Read the model definition and answer for the solid it produces. Units are mm, in the model's axes. Face numbers are marked on the shaded views. A direction names the side the tool comes from. Give positions to 0.01 mm unless a question says otherwise; leave off trailing zeros. Write each loop counter-clockwise with the first axis right and the second up, starting at its lowest first coordinate (ties: lowest second). Pieces come first, ordered by that corner, then holes. Notation, with made-up numbers: M -14.75,56 L 23.25,56 A29 ccw 23.25,89 Z; hole C 83.5,14.5 d2. An arc over 180 degrees is marked long. Put each result on its own line as item: value.
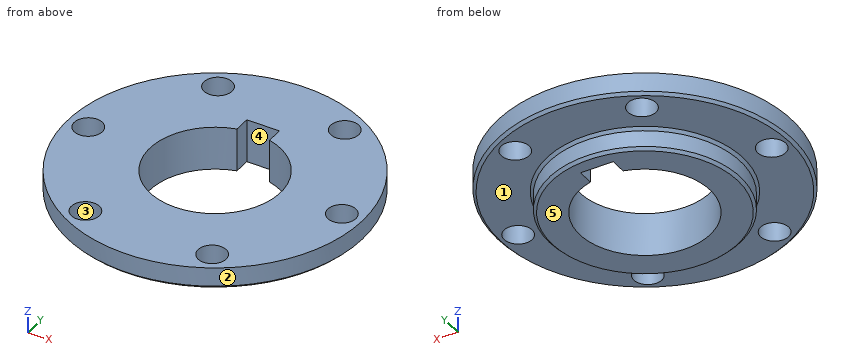
from build123d import *

# Parameters (mm, degrees)
SKETCH1_R           = 42.9895
BOSS_EXTRUDE1_DEPTH = 12.7
SKETCH2_R           = 4.1021
CUT_EXTRUDE1_DEPTH  = 13.7
SKETCH3_OUTSIDE_W   = 112.43
SKETCH3_OUTSIDE_H   = 112.43
SKETCH3_OUTSIDE_R   = 27.882207728
CUT_EXTRUDE2_DEPTH  = 6.35
CHAMFER1_SIZE       = 0.79375
CHAMFER2_SIZE       = 0.79375


with BuildPart() as part:
    # Sketch1 → Boss-Extrude1 (new body)
    with BuildSketch(Plane.XY):
        Circle(SKETCH1_R)
        with BuildLine():
            Line((-4.7625, 23.207583186), (-4.7625, 18.445083186))
            ThreePointArc((-4.7625, 18.445083186), (0, -19.05), (4.7625, 18.445083186))
            Line((4.7625, 18.445083186), (4.7625, 23.207583186))
            Line((4.7625, 23.207583186), (-4.7625, 23.207583186))
        make_face(mode=Mode.SUBTRACT)
    extrude(amount=BOSS_EXTRUDE1_DEPTH)

    # Sketch2 → Cut-Extrude1 (cut, through all)
    with BuildSketch(Plane.XY):
        with Locations((36.9951, 0)):
            Circle(SKETCH2_R)
        with Locations((18.49755, -32.038696425)):
            Circle(SKETCH2_R)
        with Locations((-18.49755, -32.038696425)):
            Circle(SKETCH2_R)
        with Locations((-36.9951, 0)):
            Circle(SKETCH2_R)
        with Locations((-18.49755, 32.038696425)):
            Circle(SKETCH2_R)
        with Locations((18.49755, 32.038696425)):
            Circle(SKETCH2_R)
    extrude(amount=CUT_EXTRUDE1_DEPTH, mode=Mode.SUBTRACT)

    # Sketch3 outside → Cut-Extrude2 (cut)
    with BuildSketch(Plane.XY):
        Rectangle(SKETCH3_OUTSIDE_W, SKETCH3_OUTSIDE_H)
        Circle(SKETCH3_OUTSIDE_R, mode=Mode.SUBTRACT)
    extrude(amount=CUT_EXTRUDE2_DEPTH, mode=Mode.SUBTRACT)

    # Chamfer1
    chamfer1_edges = [part.edges().sort_by_distance(p)[0] for p in [
        (-42.9895, 0, 6.35),
        (-27.882207728, 0, 0),
    ]]
    chamfer(chamfer1_edges, length=CHAMFER1_SIZE)

    # Chamfer2
    chamfer2_edges = [part.edges().sort_by_distance(p)[0] for p in [
        (-27.882207728, 0, 6.35),
    ]]
    chamfer(chamfer2_edges, length=CHAMFER2_SIZE)


solid = part.part
(1) Straight lines are drawn through the part: line 1 along X through (y, z) = (0, 11); line 2 along X through (y, z) = (-2.5, 8.25); line 3 along X through (y, z) = (31.5, 10). For each, find the intervals that lie inside material, in ascending order. Write a range as from..to.
Result:
line 1: x = -42.99..-41.1, -32.89..-19.05, 19.05..32.89, 41.1..42.99
line 2: x = -42.92..-40.25, -33.74..-18.89, 18.89..33.74, 40.25..42.92
line 3: x = -29.25..-22.56, -14.43..14.43, 22.56..29.25
(2) Which of the six approach directions +Z, -Z, +X, -X, +Y, -Y give full straight-line access (tool end or side, diameter ignored) to the marked faces 4 and 5?
Result:
face 4: +Z, -Z
face 5: -Z, +X, -X, +Y, -Y
(3) Section B-B on y = 0 is taken. Determine the outline of the cut face in (x, z), and give its area (3 significant figures).
Result:
outline: M -42.99,7.14 L -42.2,6.35 L -41.1,6.35 L -41.1,12.7 L -42.99,12.7 Z; M -32.89,6.35 L -28.68,6.35 L -27.88,5.56 L -27.88,0.79 L -27.09,0 L -19.05,0 L -19.05,12.7 L -32.89,12.7 Z; M 19.05,0 L 27.09,0 L 27.88,0.79 L 27.88,5.56 L 28.68,6.35 L 32.89,6.35 L 32.89,12.7 L 19.05,12.7 Z; M 41.1,6.35 L 42.2,6.35 L 42.99,7.14 L 42.99,12.7 L 41.1,12.7 Z
area: 311 mm²
(4) For a pull along Y with two mould halves and no side action, classify the marked faces 1, 2 and 3 as +Y half, -Y half, draft (parallel to the pull), parting line (faces both ways), or undercut.
Result:
face 1: draft
face 2: parting line
face 3: undercut
(5) Given pin 1 Ø1 at (y, z) = (19, 10) entering from -X; pin 2 Ø7.5 at (x, z) = (2.5, 3.5) entering from -Y; pin 3 Ø10.5 at (x, y) = (37, 0) entering from -Z, each flat-ended and moving along its own axis, determine where each tip first touches the part or whether it passes through.
Result:
pin 1: stops at x = -38.81
pin 2: stops at y = -42.96
pin 3: stops at z = 6.35
(6) Section C-C on x = -17 is taken. Give the number of separate pieces and of enclosed holes in the cut face, and give its area (3 significant figures).
Result:
separate pieces: 4
enclosed holes: 0
area: 466 mm²
(7) Section A-A on x = 0 is taken. Determine the outline of the cut face in (y, z).
Result:
outline: M -42.99,7.14 L -42.2,6.35 L -28.68,6.35 L -27.88,5.56 L -27.88,0.79 L -27.09,0 L -19.05,0 L -19.05,12.7 L -42.99,12.7 Z; M 23.21,0 L 27.09,0 L 27.88,0.79 L 27.88,5.56 L 28.68,6.35 L 42.2,6.35 L 42.99,7.14 L 42.99,12.7 L 23.21,12.7 Z
